The model under review builds one solid part; all positions refer to its coordinate system, in mm. Face numbers are marked on the shaded views. A direction names the side the tool comes from. Coordinates: 2 decimals unless noted, no trailing zeros. Order: outer loops, then holes, each group sorted by start corner. A loop starts at its lowest first (then second) coordinate and runs counter-clockwise, first axis right, second up.
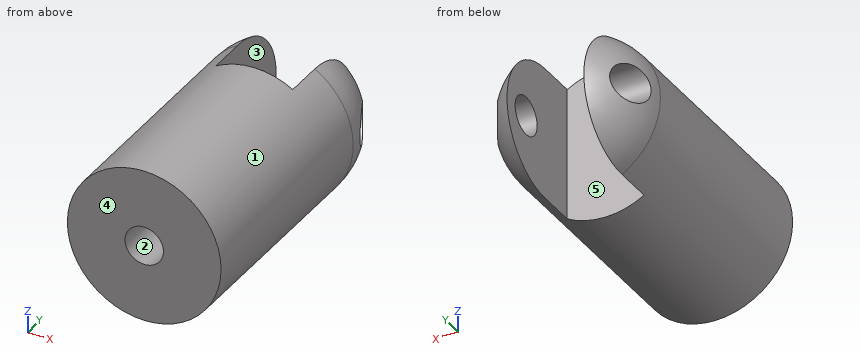
```python
from build123d import *

# Parameters (mm, degrees)
SKETCH2_W          = 25.4
SKETCH2_H          = 38.1
CUT_EXTRUDE1_DEPTH = 101.6
SKETCH3_R          = 6.35
CUT_EXTRUDE2_DEPTH = 101.6
SKETCH4_R          = 6.35
CUT_EXTRUDE3_DEPTH = 25.4


with BuildPart() as part:
    # Sketch1 → Revolve3 (revolve)
    with BuildSketch(Plane.XY):
        with BuildLine():
            Line((0, -50.8), (0, 50.8))
            ThreePointArc((0, 50.8), (17.960512242, 43.360512242), (25.4, 25.4))
            Line((25.4, 25.4), (25.4, -50.8))
            Line((25.4, -50.8), (0, -50.8))
        make_face()
    revolve(axis=Axis((0, -50.8, 0), (0, 1, 0)))

    # Sketch2 → Cut-Extrude1 (cut, symmetric)
    with BuildSketch(Plane.XY):
        with Locations((0, 31.75)):
            Rectangle(SKETCH2_W, SKETCH2_H)
    extrude(amount=CUT_EXTRUDE1_DEPTH, both=True, mode=Mode.SUBTRACT)

    # Sketch3 → Cut-Extrude2 (cut, symmetric)
    with BuildSketch(Plane(origin=(-12.7, 0, 0), x_dir=(0, 0, -1), z_dir=(1, 0, 0))):
        with Locations((0, 36.398522628)):
            Circle(SKETCH3_R)
    extrude(amount=CUT_EXTRUDE2_DEPTH, both=True, mode=Mode.SUBTRACT)

    # Sketch4 → Cut-Extrude3 (cut)
    with BuildSketch(Plane.XZ.offset(50.8)):
        Circle(SKETCH4_R)
    extrude(amount=-CUT_EXTRUDE3_DEPTH, mode=Mode.SUBTRACT)


solid = part.part
```
(1) Draft analysis for pull direction Z (two halves, no side actions). For the marked faces 1, 2 and 3, state which applies: released by +Z, released by -Z, zero draft, split by the parting line, or undercut.
A:
face 1: split by the parting line
face 2: undercut
face 3: zero draft
(2) We need section A-A, the plane x = 0. Write out the cut boundary in (y, z), and give its area (3 significant figures).
A:
outline: (-50.8, -25.4) - (12.7, -25.4) - (12.7, 25.4) - (-50.8, 25.4) - (-50.8, 6.35) - (-25.4, 6.35) - (-25.4, -6.35) - (-50.8, -6.35) - close
area: 2,900 mm2
(3) Wall thickness on probe 1 along Z at (x, y) = (-0.5, -36); probe 2 along Y at (x, z) = (-21, 0.5); probe 3 along Y at (x, z) = (-5.5, 20): over which ranges is each line inside the solid? List them lowest first.
A:
probe 1: z = -25.4 to -6.33, 6.33 to 25.4
probe 2: y = -50.8 to 30.07
probe 3: y = -50.8 to 12.7
(4) We need section B-B, the plane z = 0. Write out the cut boundary in (x, y), and give its area (3 significant figures).
A:
outline: (-25.4, -50.8) - (-6.35, -50.8) - (-6.35, -25.4) - (6.35, -25.4) - (6.35, -50.8) - (25.4, -50.8) - (25.4, 25.4) arc R25.4 ccw to (24.97, 30.05) - (12.7, 30.05) - (12.7, 12.7) - (-12.7, 12.7) - (-12.7, 30.05) - (-24.97, 30.05) arc R25.4 ccw to (-25.4, 25.4) - close; (-18.55, 42.75) - (-12.7, 42.75) - (-12.7, 47.4) arc R25.4 ccw to start; (12.7, 42.75) - (18.55, 42.75) arc R25.4 ccw to (12.7, 47.4) - close
area: 3,370 mm2
(5) Machinability: for the marked faces 4 and 5, which of the approach directions +Z, -Z, +X, -X, +Y, -Y give a long, thin tool a straight path to every point of the face, cutting with its end or side? Answer none if there is none.
A:
face 4: +Z, -Z, +X, -X, -Y
face 5: +Z, -Z, +Y
(6) We need section D-D, the plane y = 3. Write out the cut boundary in (x, z).
A:
outline: circle Ø50.8 at (0, 0)
(7) We need section C-C, the plane z = 21. Write out the cut boundary in (x, y).
A:
outline: (-14.29, -50.8) - (14.29, -50.8) - (14.29, 25.4) arc R14.29 ccw to (12.7, 31.95) - (12.7, 12.7) - (-12.7, 12.7) - (-12.7, 31.95) arc R14.29 ccw to (-14.29, 25.4) - close
(8) For pin 1 Ø16.5 at (y, z) = (36.4, 0) entering from -X; pin 2 Ø4 at (x, y) = (14, -34.5) entering from -Z; pin 3 Ø1.5 at (x, z) = (-5, -11.5) entering from +Y, all flat-tipped, find the tip position at first contact; note any pin that passes through.
A:
pin 1: stops at x = -25.25
pin 2: stops at z = -22.39
pin 3: stops at y = 12.7
